from build123d import *

# Parameters (mm, degrees)
F1_DEPTH = 50.8
F2_R     = 21.706798
F3_R     = 21.320862
F5_DEPTH = 157.70323
F7_DEPTH = 29.04742


with BuildPart() as f1:
    # F0 (on Top) → F1 (new body)
    with BuildSketch(Plane.XY):
        Polygon((68.056519, -16.868673), (68.056519, 21.231327), (36.306519, 21.231327), (8.058664, 63.453343), (-50.361336, 63.453343), (-50.361336, -59.09069), (8.058664, -59.09069), (36.306519, -16.868673), align=None)
    extrude(amount=F1_DEPTH)

    # F2
    f2_edges = [f1.edges().sort_by_distance(p)[0] for p in [
        (-50.361336, 2.181327, 0),
    ]]
    fillet(f2_edges, radius=F2_R)

    # F3
    f3_edges = [f1.edges().sort_by_distance(p)[0] for p in [
        (-50.361336, 2.181327, 50.8),
    ]]
    fillet(f3_edges, radius=F3_R)

    # F4 (on face) → F5 (cut)
    with BuildSketch(Plane.XZ.offset(59.09069)):
        with BuildLine():
            Line((99.388748, 38.1), (8.058664, 38.1))
            Line((8.058664, 38.1), (-24.523535, 38.1))
            ThreePointArc((-24.523535, 38.1), (-29.013663, 36.240128), (-30.873535, 31.75))
            Line((-30.873535, 31.75), (-30.873535, 19.05))
            ThreePointArc((-30.873535, 19.05), (-29.013663, 14.559872), (-24.523535, 12.7))
            Line((-24.523535, 12.7), (8.058664, 12.7))
            Line((8.058664, 12.7), (99.388748, 12.7))
            Line((99.388748, 12.7), (99.388748, 38.1))
        make_face()
        with BuildLine():
            Line((8.058664, 12.7), (8.058664, 38.1))
            Line((8.058664, 38.1), (-24.523535, 38.1))
            ThreePointArc((-24.523535, 38.1), (-29.013663, 36.240128), (-30.873535, 31.75))
            Line((-30.873535, 31.75), (-30.873535, 19.05))
            ThreePointArc((-30.873535, 19.05), (-29.013663, 14.559872), (-24.523535, 12.7))
            Line((-24.523535, 12.7), (8.058664, 12.7))
        make_face()
    extrude(amount=-F5_DEPTH, mode=Mode.SUBTRACT)

    # F6 (on face) → F7 (join)
    with BuildSketch(Plane.XY.offset(12.7)):
        Polygon((19.727962, 4.946723), (19.727962, 0.592731), (30.337321, -0.358673), (30.337321, 4.721327), align=None)
    extrude(amount=F7_DEPTH)


solid = f1.part
Could you check a few things on this model? Use its own coordinates, in mm. A direction names the side the tool comes from. Give positions to 0.01 mm unless a question says otherwise; leave off trailing zeros. Order: outer loops, then holes, each group sorted by start corner. A loop starts at its lowest first (then second) coordinate and runs counter-clockwise, first axis right, second up.
Item 1: For faces 1 (the face through (52, -16.869, 44)), 2 (the face through (52, 21.231, 44)), 3 (the face through (68.057, 2, 6)), which set-ups out of +Z, -Z, +X, -X, +Y, -Y let a thin tool reach every point of the face, with its end or its side?
Item 2: If we mould it in two halves opening along Z, with no side actions, what happens to faces 4 (the face through (52, 21.231, 6)), 5 (the face through (8, 3, 50.8)), 6 (the face through (19.728, 3, 25))? For each: pulls with the +Z half, pulls with the -Z half, needs draft (parallel to the pull), parting line crosses it, or undercut.
Item 3: I need wall thicknesses on line 1 (Z direction, x = -4.5, y = 0); line 2 (Z direction, x = -28, y = 18); line 3 (Y direction, x = 49.5, z = 44.5). Which ranges of each line are inside material? Lowest first, please.
Item 4: If we section it at C-C, the plane y = 17: Write out the boundary of the cut face in (x, z).
Item 5: If we section it at D-D, the plane x = 45.5: Write out the boundary of the cut face in (y, z), plus the area to 3 significant figures.
Item 6: If we section it at B-B, the plane z = 7.5: Write out the boundary of the cut face in (x, y).
Item 7: I'm going to push flat-ended pins straight in: pin 1 (12 mm diameter, centred on y = 5.5, z = 36.5, fed in from -X); pin 2 (10 mm diameter, centred on y = 28.5, z = 23, fed in from +X); pin 3 (10 mm diameter, centred on x = 40.5, z = 13, fed in from +Y). Where does each tip first touch, or does it pass through?
Item 8: If we section it at A-A, the plane x = -19.5: Write out the boundary of the cut face in (y, z), plus the area to 3 significant figures.
Values:
1. face 1: +Z, -Z, +X, -Y
1. face 2: +Z, -Z, +X, +Y
1. face 3: +Z, -Z, +X, +Y, -Y
2. face 4: needs draft
2. face 5: pulls with the +Z half
2. face 6: undercut
3. line 1: z = 0 to 12.7, 38.1 to 50.8
3. line 2: z = 0 to 13.74, 37.06 to 50.8
3. line 3: y = -16.87 to 21.23
4. outline: (-50.36, 21.71) arc R21.71 ccw to (-28.65, 0) - (68.06, 0) - (68.06, 12.7) - (-24.52, 12.7) arc R6.35 cw to (-30.87, 19.05) - (-30.87, 31.75) arc R6.35 cw to (-24.52, 38.1) - (68.06, 38.1) - (68.06, 50.8) - (-29.04, 50.8) arc R21.32 ccw to (-50.36, 29.48) - close
5. outline: (-16.87, 0) - (21.23, 0) - (21.23, 12.7) - (-16.87, 12.7) - close; (-16.87, 38.1) - (21.23, 38.1) - (21.23, 50.8) - (-16.87, 50.8) - close
5. area: 968 mm2
6. outline: (-45.07, -59.09) - (8.06, -59.09) - (36.31, -16.87) - (68.06, -16.87) - (68.06, 21.23) - (36.31, 21.23) - (8.06, 63.45) - (-45.07, 63.45) - close
7. pin 1: stops at x = -50.34
7. pin 2: stops at x = -30.79
7. pin 3: stops at y = 22.42
8. outline: (-59.09, 0) - (63.45, 0) - (63.45, 12.7) - (-59.09, 12.7) - close; (-59.09, 38.1) - (63.45, 38.1) - (63.45, 50.8) - (-59.09, 50.8) - close
8. area: 3,110 mm2
